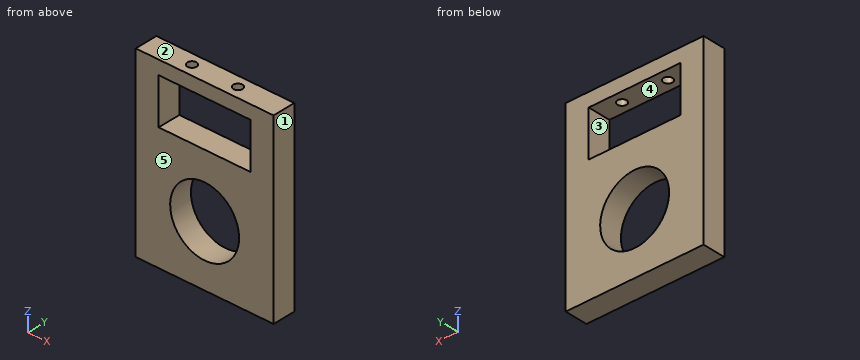
from build123d import *

# Parameters (mm, degrees)
SKETCH1_W           = 60
SKETCH1_H           = 80
BOSS_EXTRUDE1_DEPTH = 10
SKETCH2_R           = 15
CUT_EXTRUDE1_DEPTH  = 80
SKETCH3_W           = 40
SKETCH3_H           = 20
CUT_EXTRUDE2_DEPTH  = 80
SKETCH4_R           = 2
CUT_EXTRUDE3_DEPTH  = 10


with BuildPart() as part:
    # Sketch1 → Boss-Extrude1 (new body)
    with BuildSketch(Plane(origin=(0, 0, 0), x_dir=(1, 0, 0), z_dir=(0, 1, 0))):
        Rectangle(SKETCH1_W, SKETCH1_H)
    extrude(amount=BOSS_EXTRUDE1_DEPTH)

    # Sketch2 → Cut-Extrude1 (cut)
    with BuildSketch(Plane(origin=(0, 10, 0), x_dir=(1, 0, 0), z_dir=(0, 1, 0))):
        with Locations(Location((0, 13.5, 0), (0, 0, 270))):
            Circle(SKETCH2_R)
    extrude(amount=-CUT_EXTRUDE1_DEPTH, mode=Mode.SUBTRACT)

    # Sketch3 → Cut-Extrude2 (cut)
    with BuildSketch(Plane(origin=(0, 10, 0), x_dir=(1, 0, 0), z_dir=(0, 1, 0))):
        with Locations((0, -24)):
            Rectangle(SKETCH3_W, SKETCH3_H)
    extrude(amount=-CUT_EXTRUDE2_DEPTH, mode=Mode.SUBTRACT)

    # Sketch4 → Cut-Extrude3 (cut)
    with BuildSketch(Plane(origin=(0, 0, 34), x_dir=(-1, 0, 0), z_dir=(0, 0, -1))):
        with Locations((10, 5)):
            Circle(SKETCH4_R)
        with Locations((-10, 5)):
            Circle(SKETCH4_R)
    extrude(amount=-CUT_EXTRUDE3_DEPTH, mode=Mode.SUBTRACT)


solid = part.part
Here's how the part is built. I have some questions about the finished solid (model axes, mm). Face numbers are marked on the shaded views. A direction names the side the tool comes from. Give positions to 0.01 mm unless a question says otherwise; leave off trailing zeros. Loops run counter-clockwise (first coordinate to the right, second up) from the corner with the lowest first, then second, coordinate; pieces in that order, holes last. Notation, with made-up numbers: (-17, 35) -> (34, 35) arc R21 cw to (34, 66) -> close; hole circle Ø9 at (15.25, 15.25). An arc over 180 degrees is marked (long way). One line per item, written item: value.
Q1. I'm going to push a flat-ended pin straight in: pin 1 Ø6 at (x, z) = (-0.5, -4) entering from +Y. Where does the tip first touch, or does it pass through?
Answers follow:
pin 1: through
Q2. Suppose I cut it at A-A on x = 0. Please give me the cut outline in (y, z), then the cut area to 3 significant figures.
Answers follow:
outline: (0, -40) -> (10, -40) -> (10, -28.5) -> (0, -28.5) -> close; (0, 1.5) -> (10, 1.5) -> (10, 14) -> (0, 14) -> close; (0, 34) -> (10, 34) -> (10, 40) -> (0, 40) -> close
area: 300 mm^2
Q3. Suppose I cut it at B-B on y = 5. Please give me the cut outline in (x, z), then the cut area to 3 significant figures.
Answers follow:
outline: (-30, -40) -> (30, -40) -> (30, 40) -> (12, 40) -> (12, 34) -> (20, 34) -> (20, 14) -> (-20, 14) -> (-20, 34) -> (-12, 34) -> (-12, 40) -> (-30, 40) -> close; (-8, 34) -> (8, 34) -> (8, 40) -> (-8, 40) -> close; hole circle Ø30 at (0, -13.5)
area: 3,250 mm^2
Q4. On a 3-axis mill with a long thin cutter (end or side, diameter ignored), from which of +Z, -Z, +X, -X, +Y, -Y can I reach the whole of each face in a straight line? I mean the marked faces 4 and 5. Say none if no direction works.
Answers follow:
face 4: +Y, -Y
face 5: +Z, -Z, +X, -X, -Y
Q5. We'd pull the mould along Z, two halves only. Please class the marked faces 1, 2 and 3: pulls with the +Z half, pulls with the -Z half, needs draft (parallel to the pull), parting line crosses it, or undercut.
Answers follow:
face 1: needs draft
face 2: pulls with the +Z half
face 3: undercut
Q6. Suppose I cut it at C-C on z = 26.5. Please give me the cut outline in (x, y).
Answers follow:
outline: (-30, 0) -> (-20, 0) -> (-20, 10) -> (-30, 10) -> close; (20, 0) -> (30, 0) -> (30, 10) -> (20, 10) -> close
Q7. If I drill on line 1 along Y through (x, z) = (-10, 38); line 2 along Z through (x, y) = (-13, 3.5); line 3 along Z through (x, y) = (-15.5, 8.75), over which ranges is the centre line in solid material (lowest first)?
Answers follow:
line 1: 0 to 3, 7 to 10
line 2: -40 to -20.98, -6.02 to 14, 34 to 40
line 3: -40 to 14, 34 to 40
Q8. Suppose I cut it at D-D on x = -10. Please give me the cut outline in (y, z).
Answers follow:
outline: (0, -40) -> (10, -40) -> (10, -24.68) -> (0, -24.68) -> close; (0, -2.32) -> (10, -2.32) -> (10, 14) -> (0, 14) -> close; (0, 34) -> (3, 34) -> (3, 40) -> (0, 40) -> close; (7, 34) -> (10, 34) -> (10, 40) -> (7, 40) -> close
